```python
from build123d import *

# Parameters (mm, degrees)
SKETCH1_W           = 190.5
SKETCH1_H           = 76.2
BOSS_EXTRUDE1_DEPTH = 6.35
SKETCH2_W           = 6.35
SKETCH2_H           = 50.8
BOSS_EXTRUDE2_DEPTH = 6.35
SKETCH3_W           = 6.35
SKETCH3_H           = 50.8
BOSS_EXTRUDE3_DEPTH = 6.35
SKETCH4_W           = 38.1
SKETCH4_H           = 6.35
BOSS_EXTRUDE4_DEPTH = 6.35
CUT_EXTRUDE1_REACH  = 8.35
SKETCH7_R           = 3
SKETCH7_R_2         = 3.5
SKETCH7_W           = 1
SKETCH7_H           = 3
SKETCH8_R           = 1.524
CUT_EXTRUDE2_DEPTH  = 6.35


with BuildPart() as part:
    # Sketch1 → Boss-Extrude1 (new body)
    with BuildSketch(Plane.XY):
        Rectangle(SKETCH1_W, SKETCH1_H)
    extrude(amount=BOSS_EXTRUDE1_DEPTH)

    # Sketch2 → Boss-Extrude2 (add)
    with BuildSketch(Plane.ZY.offset(95.25)):
        with Locations((3.175, 0)):
            Rectangle(SKETCH2_W, SKETCH2_H)
    extrude(amount=BOSS_EXTRUDE2_DEPTH)

    # Sketch3 → Boss-Extrude3 (add)
    with BuildSketch(Plane(origin=(95.25, 0, 0), x_dir=(0, 0, -1), z_dir=(1, 0, 0))):
        with Locations((-3.175, 0)):
            Rectangle(SKETCH3_W, SKETCH3_H)
    extrude(amount=BOSS_EXTRUDE3_DEPTH)

    # Sketch4 → Boss-Extrude4 (add)
    with BuildSketch(Plane.XZ.offset(38.1)):
        with Locations((-50.8, 3.175)):
            Rectangle(SKETCH4_W, SKETCH4_H)
        with Locations((50.8, 3.175)):
            Rectangle(SKETCH4_W, SKETCH4_H)
    extrude(amount=BOSS_EXTRUDE4_DEPTH)

    # Sketch7 → Cut-Extrude1 (cut, up to next)
    with BuildSketch(Plane(origin=(0, 0, 0), x_dir=(-1, 0, 0), z_dir=(0, 0, -1)), mode=Mode.PRIVATE) as cut_extrude1_sk1:
        with Locations((-30.48, 15.24)):
            Circle(SKETCH7_R)
    cut_extrude1_tool1 = extrude(cut_extrude1_sk1.sketch, amount=-CUT_EXTRUDE1_REACH, mode=Mode.PRIVATE) & part.part
    add(cut_extrude1_tool1.solids().sort_by_distance((30.48, 15.24, 0))[0], mode=Mode.SUBTRACT)
    # Sketch7 → Cut-Extrude1 (cut, up to next)
    with BuildSketch(Plane(origin=(0, 0, 0), x_dir=(-1, 0, 0), z_dir=(0, 0, -1)), mode=Mode.PRIVATE) as cut_extrude1_sk2:
        with Locations((0, 15.24)):
            Circle(SKETCH7_R)
    cut_extrude1_tool2 = extrude(cut_extrude1_sk2.sketch, amount=-CUT_EXTRUDE1_REACH, mode=Mode.PRIVATE) & part.part
    add(cut_extrude1_tool2.solids().sort_by_distance((0, 15.24, 0))[0], mode=Mode.SUBTRACT)
    # Sketch7 → Cut-Extrude1 (cut, up to next)
    with BuildSketch(Plane(origin=(0, 0, 0), x_dir=(-1, 0, 0), z_dir=(0, 0, -1)), mode=Mode.PRIVATE) as cut_extrude1_sk3:
        with Locations((30.48, 15.24)):
            Circle(SKETCH7_R)
    cut_extrude1_tool3 = extrude(cut_extrude1_sk3.sketch, amount=-CUT_EXTRUDE1_REACH, mode=Mode.PRIVATE) & part.part
    add(cut_extrude1_tool3.solids().sort_by_distance((-30.48, 15.24, 0))[0], mode=Mode.SUBTRACT)
    # Sketch7 → Cut-Extrude1 (cut, up to next)
    with BuildSketch(Plane(origin=(0, 0, 0), x_dir=(-1, 0, 0), z_dir=(0, 0, -1)), mode=Mode.PRIVATE) as cut_extrude1_sk4:
        with Locations((60.96, 15.24)):
            Circle(SKETCH7_R)
    cut_extrude1_tool4 = extrude(cut_extrude1_sk4.sketch, amount=-CUT_EXTRUDE1_REACH, mode=Mode.PRIVATE) & part.part
    add(cut_extrude1_tool4.solids().sort_by_distance((-60.96, 15.24, 0))[0], mode=Mode.SUBTRACT)
    # Sketch7 → Cut-Extrude1 (cut, up to next)
    with BuildSketch(Plane(origin=(0, 0, 0), x_dir=(-1, 0, 0), z_dir=(0, 0, -1)), mode=Mode.PRIVATE) as cut_extrude1_sk5:
        with Locations((0, -15.24)):
            Circle(SKETCH7_R)
    cut_extrude1_tool5 = extrude(cut_extrude1_sk5.sketch, amount=-CUT_EXTRUDE1_REACH, mode=Mode.PRIVATE) & part.part
    add(cut_extrude1_tool5.solids().sort_by_distance((0, -15.24, 0))[0], mode=Mode.SUBTRACT)
    # Sketch7 → Cut-Extrude1 (cut, up to next)
    with BuildSketch(Plane(origin=(0, 0, 0), x_dir=(-1, 0, 0), z_dir=(0, 0, -1)), mode=Mode.PRIVATE) as cut_extrude1_sk6:
        with Locations((30.48, -15.24)):
            Circle(SKETCH7_R)
    cut_extrude1_tool6 = extrude(cut_extrude1_sk6.sketch, amount=-CUT_EXTRUDE1_REACH, mode=Mode.PRIVATE) & part.part
    add(cut_extrude1_tool6.solids().sort_by_distance((-30.48, -15.24, 0))[0], mode=Mode.SUBTRACT)
    # Sketch7 → Cut-Extrude1 (cut, up to next)
    with BuildSketch(Plane(origin=(0, 0, 0), x_dir=(-1, 0, 0), z_dir=(0, 0, -1)), mode=Mode.PRIVATE) as cut_extrude1_sk7:
        with Locations((60.96, -15.24)):
            Circle(SKETCH7_R)
    cut_extrude1_tool7 = extrude(cut_extrude1_sk7.sketch, amount=-CUT_EXTRUDE1_REACH, mode=Mode.PRIVATE) & part.part
    add(cut_extrude1_tool7.solids().sort_by_distance((-60.96, -15.24, 0))[0], mode=Mode.SUBTRACT)
    # Sketch7 → Cut-Extrude1 (cut, up to next)
    with BuildSketch(Plane(origin=(0, 0, 0), x_dir=(-1, 0, 0), z_dir=(0, 0, -1)), mode=Mode.PRIVATE) as cut_extrude1_sk8:
        with Locations((-30.48, -15.24)):
            Circle(SKETCH7_R)
    cut_extrude1_tool8 = extrude(cut_extrude1_sk8.sketch, amount=-CUT_EXTRUDE1_REACH, mode=Mode.PRIVATE) & part.part
    add(cut_extrude1_tool8.solids().sort_by_distance((30.48, -15.24, 0))[0], mode=Mode.SUBTRACT)
    # Sketch7 → Cut-Extrude1 (cut, up to next)
    with BuildSketch(Plane(origin=(0, 0, 0), x_dir=(-1, 0, 0), z_dir=(0, 0, -1)), mode=Mode.PRIVATE) as cut_extrude1_sk9:
        with Locations((-60.96, 15.24)):
            Circle(SKETCH7_R_2)
    cut_extrude1_tool9 = extrude(cut_extrude1_sk9.sketch, amount=-CUT_EXTRUDE1_REACH, mode=Mode.PRIVATE) & part.part
    add(cut_extrude1_tool9.solids().sort_by_distance((60.96, 15.24, 0))[0], mode=Mode.SUBTRACT)
    # Sketch7 → Cut-Extrude1 (cut, up to next)
    with BuildSketch(Plane(origin=(0, 0, 0), x_dir=(-1, 0, 0), z_dir=(0, 0, -1)), mode=Mode.PRIVATE) as cut_extrude1_sk10:
        with Locations((-60.96, -15.24)):
            Circle(SKETCH7_R_2)
    cut_extrude1_tool10 = extrude(cut_extrude1_sk10.sketch, amount=-CUT_EXTRUDE1_REACH, mode=Mode.PRIVATE) & part.part
    add(cut_extrude1_tool10.solids().sort_by_distance((60.96, -15.24, 0))[0], mode=Mode.SUBTRACT)
    # Sketch7 → Cut-Extrude1 (cut, up to next)
    with BuildSketch(Plane(origin=(0, 0, 0), x_dir=(-1, 0, 0), z_dir=(0, 0, -1)), mode=Mode.PRIVATE) as cut_extrude1_sk11:
        with Locations((-68.96, 15.24)):
            Rectangle(SKETCH7_W, SKETCH7_H)
    cut_extrude1_tool11 = extrude(cut_extrude1_sk11.sketch, amount=-CUT_EXTRUDE1_REACH, mode=Mode.PRIVATE) & part.part
    add(cut_extrude1_tool11.solids().sort_by_distance((68.96, 15.24, 0))[0], mode=Mode.SUBTRACT)
    # Sketch7 → Cut-Extrude1 (cut, up to next)
    with BuildSketch(Plane(origin=(0, 0, 0), x_dir=(-1, 0, 0), z_dir=(0, 0, -1)), mode=Mode.PRIVATE) as cut_extrude1_sk12:
        with Locations((-68.96, -15.24)):
            Rectangle(SKETCH7_W, SKETCH7_H)
    cut_extrude1_tool12 = extrude(cut_extrude1_sk12.sketch, amount=-CUT_EXTRUDE1_REACH, mode=Mode.PRIVATE) & part.part
    add(cut_extrude1_tool12.solids().sort_by_distance((68.96, -15.24, 0))[0], mode=Mode.SUBTRACT)

    # Sketch8 → Cut-Extrude2 (cut)
    with BuildSketch(Plane(origin=(23.763692911, 98.5857123, 6.35), x_dir=(1, 0, 0), z_dir=(0, 0, 1))):
        with Locations((-109.488692911, -120.8107123)):
            Circle(SKETCH8_R)
        with Locations((61.961307089, -120.8107123)):
            Circle(SKETCH8_R)
    extrude(amount=-CUT_EXTRUDE2_DEPTH, mode=Mode.SUBTRACT)


solid = part.part
```
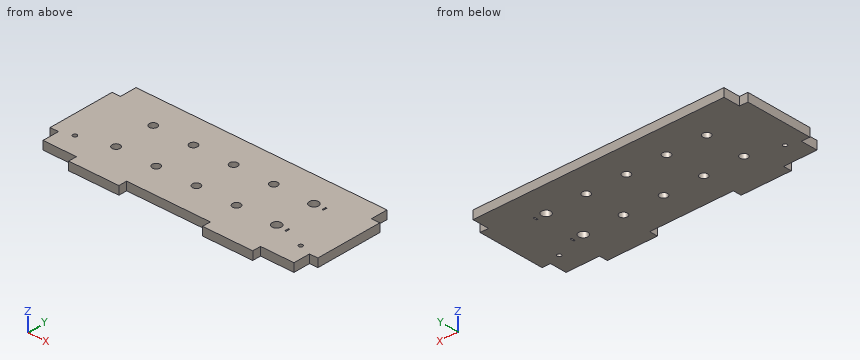
CAD build for the part. Positions are in the model's coordinates, mm. Round coordinates to 2 decimals unless told otherwise and drop trailing zeros. Write each loop counter-clockwise with the first axis right and the second up, starting at its lowest first coordinate (ties: lowest second). Pieces come first, ordered by that corner, then holes. Notation, with made-up numbers: (-38.75, 48.5) - (10.25, 48.5) arc R17 ccw to (10.25, 76.5) - close; hole circle Ø2 at (88.5, -10.5). An arc over 180 degrees is marked (long way). Return JSON: item names as keys, results as strings. Group by question number.
Item 1: Band-saw the part on B-B on x = 0. List the corners of the cut face in (y, z), plus the area to 3 significant figures.
Item 2: Band-saw the part on A-A on x = 60.96. List the corners of the cut face in (y, z).
Item 3: Band-saw the part on C-C on y = 30.5. List the corners of the cut face in (x, z).
Item 4: Band-saw the part on D-D on z = 2.25. State how many separate pieces and enclosed holes the cut face has, plus the area to 3 significant figures.
Item 5: Probe probe 1 along Y at (x, z) = (0, 5.25); probe 2 along Y at (x, z) = (60.96, 2.25); probe 3 along Y at (x, z) = (85.5, 0.75). List the from-to ranges inside material, lowest first.
Item 6: Flat gauge pins, fed straight in: pin 1 Ø1.5 at (x, z) = (-13, 3) entering from -Y; pin 2 Ø1.9 at (y, z) = (-31.5, 3) entering from -X; pin 3 Ø1.9 at (x, z) = (98, 2) entering from -Y. Where does each tip first touch, or does it go through?
Resolved:
{
 "1": {"outline": "(-38.1, 0) - (-18.24, 0) - (-18.24, 6.35) - (-38.1, 6.35) - close; (-12.24, 0) - (12.24, 0) - (12.24, 6.35) - (-12.24, 6.35) - close; (18.24, 0) - (38.1, 0) - (38.1, 6.35) - (18.24, 6.35) - close", "area": "408 mm²"},
 "2": {"outline": "(-44.45, 0) - (-18.74, 0) - (-18.74, 6.35) - (-44.45, 6.35) - close; (-11.74, 0) - (11.74, 0) - (11.74, 6.35) - (-11.74, 6.35) - close; (18.74, 0) - (38.1, 0) - (38.1, 6.35) - (18.74, 6.35) - close"},
 "3": {"outline": "(-95.25, 0) - (95.25, 0) - (95.25, 6.35) - (-95.25, 6.35) - close"},
 "4": {"separate pieces": "1", "enclosed holes": "14", "area": "15,300 mm²"},
 "5": {"probe 1": "y = -38.1 to -18.24, -12.24 to 12.24, 18.24 to 38.1", "probe 2": "y = -44.45 to -18.74, -11.74 to 11.74, 18.74 to 38.1", "probe 3": "y = -38.1 to -23.73, -20.72 to 38.1"},
 "6": {"pin 1": "stops at y = -38.1", "pin 2": "stops at x = -95.25", "pin 3": "stops at y = -25.4"}
}
